Read the model definition and answer for the solid it produces. Units are mm, in the model's axes. Face numbers are marked on the shaded views. A direction names the side the tool comes from. Give positions to 0.01 mm unless a question says otherwise; leave off trailing zeros. Write each loop counter-clockwise with the first axis right and the second up, starting at its lowest first coordinate (ties: lowest second). Pieces come first, ordered by that corner, then holes. Notation, with made-up numbers: M -27.75,-25.5 L 30.25,-25.5 A17 cw 30.25,-12.5 Z; hole C 29,-40 d11. An arc over 180 degrees is marked long. Use a Markdown table: item, result. Add a question column.
Item 1: The mould has two halves that part along X. Classify the marked faces 3, 4 and 5: pulls with the +X half, pulls with the -X half, needs draft (parallel to the pull), parting line crosses it, or undercut.
Item 2: A cutting plane is placed at B-B on x = 9.5. Determine the outline of the cut face in (y, z).
Item 3: A cutting plane is placed at A-A on y = 13. Determine the outline of the cut face in (x, z).
Item 4: A cutting plane is placed at C-C on z = 3.1. Determine the outline of the cut face in (x, y), then the cut area to 3 significant figures.
Item 5: Given P1, Ø1, axis at x = 17.5, z = 2.5, coming from the -Y side; P2, Ø2, axis at y = 13.5, z = 1.5, coming from the -X side; P3, Ø1.5, axis at x = 16, y = -3.5, coming from the +Z side; P4, Ø1.3, axis at x = 7.5, z = 2, coming from the +Y side, each flat-ended and moving along its own axis, determine where each tip first touches the part or whether it passes through.
Item 6: A cutting plane is placed at D-D on y = 29. Determine the outline of the cut face in (x, z), then the cut area to 3 significant figures.
Item 7: Consider probe 1 along Y at (x, z) = (13, 1.95); probe 2 along Y at (x, z) = (18, 1.7); probe 3 along X at (y, z) = (13, 1.4). Determine where each line is inside the solid, lowest interval first. Write a range as [from, to].
Item 8: For the marked faces 1 and 2, determine the directions among +Z, -Z, +X, -X, +Y, -Y from which every point of the face is accessible in a straight line to the end or side of a thin tool.
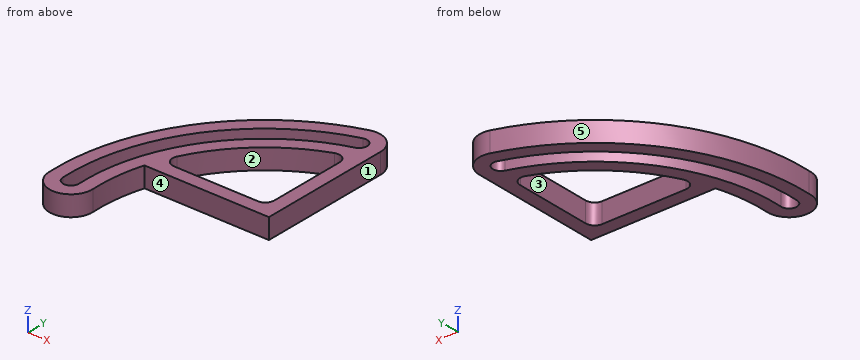
from build123d import *

# Parameters (mm, degrees)
BOSS_EXTRUDE1_DEPTH = 4.5


with BuildPart() as part:
    # Sketch1 → Boss-Extrude1 (new body)
    with BuildSketch(Plane.XY):
        with BuildLine():
            Line((-2.6366524, -1.149368065), (25.121954618, -1.149368065))
            Line((25.121954618, -1.149368065), (25.121954618, 28.374931045))
            ThreePointArc((25.121954618, 28.374931045), (23.183396216, 32.203546479), (18.950040453, 32.907111548))
            ThreePointArc((18.950040453, 32.907111548), (-5.035386419, 15.47250193), (-13.605299783, -12.914517987))
            ThreePointArc((-13.605299783, -12.914517987), (-8.8972368, -18.005680822), (-4.0694524, -13.027900808))
            ThreePointArc((-4.0694524, -13.027900808), (-3.836748935, -7.030290497), (-2.6366524, -1.149368065))
        make_face()
        with BuildLine():
            Line((1.419098269, 1.850631935), (20.121954618, 1.850631935))
            ThreePointArc((20.121954618, 1.850631935), (21.53616818, 2.436418372), (22.121954618, 3.850631935))
            Line((22.121954618, 3.850631935), (22.121954618, 21.135325995))
            ThreePointArc((22.121954618, 21.135325995), (21.249580029, 22.78713135), (19.393493686, 22.997943688))
            ThreePointArc((19.393493686, 22.997943688), (7.78243837, 15.73507518), (-0.390986112, 4.745944333))
            ThreePointArc((-0.390986112, 4.745944333), (-0.288183148, 2.79674616), (1.419098269, 1.850631935))
        make_face(mode=Mode.SUBTRACT)
        with BuildLine():
            ThreePointArc((19.848091505, 30.044681757), (-2.729641043, 13.536951641), (-10.588882657, -13.30502075))
            ThreePointArc((-10.588882657, -13.30502075), (-8.766141749, -14.979122175), (-7.092040324, -13.156381267))
            ThreePointArc((-7.092040324, -13.156381267), (0.134806128, 11.525747423), (20.895817731, 26.705180334))
            ThreePointArc((20.895817731, 26.705180334), (22.041705329, 28.898794159), (19.848091505, 30.044681757))
        make_face(mode=Mode.SUBTRACT)
    extrude(amount=BOSS_EXTRUDE1_DEPTH)


solid = part.part
Filled in:
| question | item | result |
|---|---|---|
| 1 | face 3 | undercut |
| 1 | face 4 | needs draft |
| 1 | face 5 | pulls with the -X half |
| 2 | outline | M -1.15,0 L 1.85,0 L 1.85,4.5 L -1.15,4.5 Z; M 17.22,0 L 21,0 L 21,4.5 L 17.22,4.5 Z; M 25.23,0 L 28.74,0 L 28.74,4.5 L 25.23,4.5 Z |
| 3 | outline | M -6.68,0 L -3.1,0 L -3.1,4.5 L -6.68,4.5 Z; M 1.22,0 L 5.11,0 L 5.11,4.5 L 1.22,4.5 Z; M 22.12,0 L 25.12,0 L 25.12,4.5 L 22.12,4.5 Z |
| 4 | outline | M -13.61,-12.91 A4.78 ccw long -4.07,-13.03 A36.97 cw -2.64,-1.15 L 25.12,-1.15 L 25.12,28.37 A4.75 ccw 18.95,32.91 A46.5 ccw Z; hole M -10.59,-13.31 A1.75 ccw -7.09,-13.16 A40 cw 20.9,26.71 A1.75 ccw 19.85,30.04 A43.5 ccw Z; hole M -0.39,4.75 A2.01 ccw 1.42,1.85 L 20.12,1.85 A2 ccw 22.12,3.85 L 22.12,21.14 A2 ccw 19.39,23 A37 ccw Z |
| 4 | area | 547 mm² |
| 5 | P1 | y = -1.15 |
| 5 | P2 | x = -6.98 |
| 5 | P3 | through |
| 5 | P4 | y = 27.92 |
| 6 | outline | M 9.95,0 L 16.9,0 L 16.9,4.5 L 9.95,4.5 Z; M 22.01,0 L 25.08,0 L 25.08,4.5 L 22.01,4.5 Z |
| 6 | area | 45.1 mm² |
| 7 | probe 1 | [-1.15, 1.85], [19.75, 23.26], [27.24, 30.58] |
| 7 | probe 2 | [-1.15, 1.85], [22.42, 25.67], [29.42, 32.6] |
| 7 | probe 3 | [-6.68, -3.1], [1.22, 5.11], [22.12, 25.12] |
| 8 | face 1 | +Z, -Z, +X, +Y, -Y |
| 8 | face 2 | +Z, -Z |
